```python
from build123d import *

# Parameters (mm, degrees)
SKETCH1_W           = 52
SKETCH1_H           = 28.5
SKETCH1_R           = 1.6
BOSS_EXTRUDE1_DEPTH = 1.6
FILLET1_R           = 2
SKETCH2_W           = 6
SKETCH2_H           = 8
BOSS_EXTRUDE2_DEPTH = 2.6
SKETCH3_W           = 26.5
SKETCH3_H           = 18.5
BOSS_EXTRUDE3_DEPTH = 0.9
SKETCH4_W           = 19
SKETCH4_H           = 18.5
BOSS_EXTRUDE4_DEPTH = 2.4
SKETCH5_W           = 4.480247742
SKETCH5_H           = 2.767211841
SKETCH5_H_2         = 2.398250262
BOSS_EXTRUDE5_DEPTH = 2


with BuildPart() as part:
    # Sketch1 → Boss-Extrude1 (new body)
    with BuildSketch(Plane(origin=(0, 0, 0), x_dir=(1, 0, 0), z_dir=(0, 1, 0))):
        Rectangle(SKETCH1_W, SKETCH1_H)
        with Locations(Location((-23.7, 11.55, 0), (0, 0, 270))):
            Circle(SKETCH1_R, mode=Mode.SUBTRACT)
        with Locations(Location((-23.7, -11.55, 0), (0, 0, 270))):
            Circle(SKETCH1_R, mode=Mode.SUBTRACT)
        with Locations(Location((23.4, 11.55, 0), (0, 0, 270))):
            Circle(SKETCH1_R, mode=Mode.SUBTRACT)
        with Locations(Location((23.4, -11.55, 0), (0, 0, 270))):
            Circle(SKETCH1_R, mode=Mode.SUBTRACT)
    extrude(amount=BOSS_EXTRUDE1_DEPTH)

    # Fillet1
    fillet1_edges = [part.edges().sort_by_distance(p)[0] for p in [
        (-26, 0.8, -14.25),
        (26, 0.8, -14.25),
        (26, 0.8, 14.25),
        (-26, 0.8, 14.25),
    ]]
    fillet(fillet1_edges, radius=FILLET1_R)

    # Sketch2 → Boss-Extrude2 (add)
    with BuildSketch(Plane(origin=(0, 1.6, 0), x_dir=(1, 0, 0), z_dir=(0, 1, 0))):
        with Locations((-23, 0)):
            Rectangle(SKETCH2_W, SKETCH2_H)
    extrude(amount=BOSS_EXTRUDE2_DEPTH)

    # Sketch3 → Boss-Extrude3 (add)
    with BuildSketch(Plane(origin=(0, 1.6, 0), x_dir=(1, 0, 0), z_dir=(0, 1, 0))):
        with Locations((12.75, 0)):
            Rectangle(SKETCH3_W, SKETCH3_H)
    extrude(amount=BOSS_EXTRUDE3_DEPTH)

    # Sketch4 → Boss-Extrude4 (add)
    with BuildSketch(Plane(origin=(0, 2.5, 0), x_dir=(1, 0, 0), z_dir=(0, 1, 0))):
        with Locations((9, 0)):
            Rectangle(SKETCH4_W, SKETCH4_H)
    extrude(amount=BOSS_EXTRUDE4_DEPTH)

    # Sketch5 → Boss-Extrude5 (add)
    with BuildSketch(Plane(origin=(0, 1.6, 0), x_dir=(1, 0, 0), z_dir=(0, 1, 0))):
        with Locations((-23.323642657, 8.222572326)):
            Rectangle(SKETCH5_W, SKETCH5_H)
        with Locations((-23.323642657, -8.459761913)):
            Rectangle(SKETCH5_W, SKETCH5_H_2)
    extrude(amount=BOSS_EXTRUDE5_DEPTH)


solid = part.part
```
Source: CAD feature listing. Evaluate the final solid. Frame: model axes, mm. A direction names the side the tool comes from. Coordinates: 2 decimals unless noted, no trailing zeros. Write each loop counter-clockwise with the first axis right and the second up, starting at its lowest first coordinate (ties: lowest second). Pieces come first, ordered by that corner, then holes. Notation, with made-up numbers: M -18.5,13.25 L 31.5,13.25 A24 ccw 31.5,26.25 Z; hole C 67,-10.5 d5. An arc over 180 degrees is marked long. Answer as a JSON object with one key per item and string values.
1. Draft query along X for faces 4 (the flat face through (-25.564, 3, -8)), 5 (the flat face through (0, 0, 0)), 6 (the cylindrical face through (-23.219, 0.789, 13.076)), 7 (the cylindrical face through (25.4, 0.81, -13.68)). Return one class per face: released by +X, released by -X, zero draft, split by the parting line, or undercut.
Evaluation:
{"face 4": "released by -X", "face 5": "zero draft", "face 6": "undercut", "face 7": "released by +X"}
2. Cut plane A-A on x = 23.4. Output: boundary loops of the cut face in (y, z).
Evaluation:
{"outline": "M 0,-14.25 L 1.6,-14.25 L 1.6,-13.15 L 0,-13.15 Z; M 0,-9.95 L 1.6,-9.95 L 1.6,-9.25 L 2.5,-9.25 L 2.5,9.25 L 1.6,9.25 L 1.6,9.95 L 0,9.95 Z; M 0,13.15 L 1.6,13.15 L 1.6,14.25 L 0,14.25 Z"}
3. Cut plane C-C on y = 3. Output: boundary loops of the cut face in (x, z).
Evaluation:
{"outline": "M -26,-4 L -20,-4 L -20,4 L -26,4 Z; M -25.56,-9.61 L -21.08,-9.61 L -21.08,-6.84 L -25.56,-6.84 Z; M -25.56,7.26 L -21.08,7.26 L -21.08,9.66 L -25.56,9.66 Z; M -0.5,-9.25 L 18.5,-9.25 L 18.5,9.25 L -0.5,9.25 Z"}
4. Cut plane D-D on z = 3.5. Output: boundary loops of the cut face in (x, y), plus the area to 3 significant figures.
Evaluation:
{"outline": "M -26,0 L 26,0 L 26,2.5 L 18.5,2.5 L 18.5,4.9 L -0.5,4.9 L -0.5,1.6 L -20,1.6 L -20,4.2 L -26,4.2 Z", "area": "168 mm^2"}
5. Access query for faces 1 (the flat face through (-21.084, 3, 8)), 2 (the flat face through (-20, 3, 0)), 3 (the flat face through (-25.564, 3, 8)). Directions: +Z, -Z, +X, -X, +Y, -Y. A direction counts if a zero-diameter tool reaches every point of the face in a straight line with its end or side. Return the directions, or none.
Evaluation:
{"face 1": "+Z, +Y", "face 2": "+Z, -Z, +Y", "face 3": "+Z, -X, +Y"}
6. Ray query, L1, parallel to X at y = 0.75, z = -11.55; L2, parallel to X at y = 2.15, z = 1.5; L3, parallel to X at y = 3.2, z = 0. Return the intervals inside material, ascending.
Evaluation:
{"L1": "-26 to -25.3, -22.1 to 21.8, 25 to 26", "L2": "-26 to -20, -0.5 to 26", "L3": "-26 to -20, -0.5 to 18.5"}
7. Contact query for flat-ended pins moving along their axis: P1, Ø4, axis at x = -23.7, z = -11.55, coming from the -Y side; P2, Ø6, axis at x = 22.5, z = -3.5, coming from the +Y side; P3, Ø1.9, axis at y = 4, z = 1.5, coming from the +X side; P4, Ø2.5, axis at x = 23.4, z = -11.55, coming from the -Y side. Output: stop coordinate, or through.
Evaluation:
{"P1": "y = 0", "P2": "y = 2.5", "P3": "x = 18.5", "P4": "through"}
8. Cut plane B-B on z = 11.55. Output: boundary loops of the cut face in (x, y), plus the area to 3 significant figures.
Evaluation:
{"outline": "M -26,0 L -25.3,0 L -25.3,1.6 L -26,1.6 Z; M -22.1,0 L 21.8,0 L 21.8,1.6 L -22.1,1.6 Z; M 25,0 L 26,0 L 26,1.6 L 25,1.6 Z", "area": "73.0 mm^2"}
